```python
from build123d import *

# Parameters (mm, degrees)
F0_W          = 75.9948119521
F0_H          = 111.8377298117
F0_R          = 4.7655494626
F0_R_2        = 4.8016385214
F1_DEPTH      = 39.116
F2_R          = 25.2095031521
F2_R_2        = 17.6279340775
F3_DEPTH      = 50.8
F3_DEPTH_BACK = 50.8
F4_R          = 17.506739517
F5_DEPTH      = 77.978
F5_DEPTH_BACK = 76.962
F6_W          = 38.5849960148
F6_H          = 51.1202197522
F7_DEPTH      = 50.8
F7_DEPTH_BACK = 50.8


with BuildPart() as f1:
    # F0 (on Front) → F1 (new body)
    with BuildSketch(Plane.XZ):
        Rectangle(F0_W, F0_H)
        with Locations((0, -46.5174391866)):
            Circle(F0_R, mode=Mode.SUBTRACT)
        with Locations((0, 47.8884801269)):
            Circle(F0_R_2, mode=Mode.SUBTRACT)
    extrude(amount=-F1_DEPTH)

    # F2 (on Right) → F3 (join, two sides)
    with BuildSketch(Plane.YZ) as f3_sk:
        Circle(F2_R)
        Circle(F2_R_2, mode=Mode.SUBTRACT)
    extrude(amount=F3_DEPTH)
    extrude(f3_sk.sketch, amount=-F3_DEPTH_BACK)

    # F4 (on Right) → F5 (cut, two sides)
    with BuildSketch(Plane.YZ) as f5_sk:
        Circle(F4_R)
    extrude(amount=-F5_DEPTH, mode=Mode.SUBTRACT)
    extrude(f5_sk.sketch, amount=F5_DEPTH_BACK, mode=Mode.SUBTRACT)

    # F6 (on Right) → F7 (cut, two sides)
    with BuildSketch(Plane.YZ) as f7_sk:
        with Locations((-19.2924980074, 9.313e-07)):
            Rectangle(F6_W, F6_H)
    extrude(amount=-F7_DEPTH, mode=Mode.SUBTRACT)
    extrude(f7_sk.sketch, amount=F7_DEPTH_BACK, mode=Mode.SUBTRACT)


solid = f1.part
```
Read the model definition and answer for the solid it produces. Units are mm, in the model's axes. A direction names the side the tool comes from. Coordinates: 2 decimals unless noted, no trailing zeros. Loops run counter-clockwise (first coordinate to the right, second up) from the corner with the lowest first, then second, coordinate; pieces in that order, holes last. Notation, with made-up numbers: (49, 45.25) - (59, 45.25) arc R26 ccw to (59, 78.25) - close; hole circle Ø7 at (19, -24.5). An arc over 180 degrees is marked (long way). Answer in a Markdown table with one row per item.
1. Find section D-D, the plane x = -26. Write down the section's boundary in (y, z), then the cut area to 3 significant figures.
Conclusion:
| item | result |
|---|---|
| outline | (0, -55.92) - (39.12, -55.92) - (39.12, 55.92) - (0, 55.92) - (0, 17.51) arc R17.51 cw to (0, -17.51) - close |
| area | 3,890 mm² |
2. Straight lines are drawn through the part: line 1 (Z direction, x = 0, y = 24); line 2 (Z direction, x = 0, y = 10); line 3 (X direction, y = 38, z = 39). For each, find the intervals that lie inside material, in ascending order.
Conclusion:
| item | result |
|---|---|
| line 1 | z = -55.92 to -51.28, -41.75 to 43.09, 52.69 to 55.92 |
| line 2 | z = -55.92 to -51.28, -41.75 to -14.37, 14.37 to 43.09, 52.69 to 55.92 |
| line 3 | x = -38 to 38 |
3. Which of the six approach directions +Z, -Z, +X, -X, +Y, -Y give full straight-line access (tool end or side, diameter ignored) to faces 1 (the face through (44.309, 25.203, -0.554)), 2 (the face through (-44.309, 17.624, -0.388)), 3 (the face through (-37.997, 28, -1))?
Conclusion:
| item | result |
|---|---|
| face 1 | +X, +Y |
| face 2 | -X, -Y |
| face 3 | -X, +Y |
4. Given pin 1 (8 mm diameter, centred on x = 37.5, z = 1.5, fed in from -Y); pin 2 (4 mm diameter, centred on x = 9, z = -4, fed in from -Y); pin 3 (4 mm diameter, centred on y = 35, z = -10, fed in from -X); pin 4 (12 mm diameter, centred on y = 21, z = 19.5, fed in from -X), each flat-ended and moving along its own axis, determine where each tip first touches the part or whether it passes through.
Conclusion:
| item | result |
|---|---|
| pin 1 | stops at y = 16.62 |
| pin 2 | stops at y = 16.45 |
| pin 3 | stops at x = -38 |
| pin 4 | stops at x = -50.8 |
5. Find section C-C, the plane z = 0. Write down the section's boundary in (x, y).
Conclusion:
| item | result |
|---|---|
| outline | (-50.8, 17.63) - (-38, 17.63) - (-38, 17.51) - (38, 17.51) - (38, 17.63) - (50.8, 17.63) - (50.8, 25.21) - (38, 25.21) - (38, 39.12) - (-38, 39.12) - (-38, 25.21) - (-50.8, 25.21) - close |
6. Find section A-A, the plane x = 0. Write down the section's boundary in (y, z).
Conclusion:
| item | result |
|---|---|
| outline | (0, -55.92) - (39.12, -55.92) - (39.12, -51.28) - (0, -51.28) - close; (0, -41.75) - (39.12, -41.75) - (39.12, 43.09) - (0, 43.09) - (0, 17.51) arc R17.51 cw to (0, -17.51) - close; (0, 52.69) - (39.12, 52.69) - (39.12, 55.92) - (0, 55.92) - close |
7. Find section B-B, the plane y = 12.5. Write down the section's boundary in (x, z).
Conclusion:
| item | result |
|---|---|
| outline | (-50.8, -21.89) - (-38, -21.89) - (-38, -55.92) - (38, -55.92) - (38, -21.89) - (50.8, -21.89) - (50.8, -12.43) - (38, -12.43) - (38, -12.26) - (-38, -12.26) - (-38, -12.43) - (-50.8, -12.43) - close; (-50.8, 12.43) - (-38, 12.43) - (-38, 12.26) - (38, 12.26) - (38, 12.43) - (50.8, 12.43) - (50.8, 21.89) - (38, 21.89) - (38, 55.92) - (-38, 55.92) - (-38, 21.89) - (-50.8, 21.89) - close; hole circle Ø9.6 at (0, 47.89); hole circle Ø9.53 at (0, -46.52) |
8. Determine the mould class of faces 4 (the face through (-50.8, 18, 0)), 5 (the face through (-0.62, 19.284, -41.792)), 6 (the face through (44.309, 17.624, -0.388)), 7 (the face through (-1.04, 19.28, 43.2)) for opening direction X: +X half, -X half, draft (parallel to the pull), parting line (faces both ways), or undercut.
Conclusion:
| item | result |
|---|---|
| face 4 | -X half |
| face 5 | undercut |
| face 6 | draft |
| face 7 | undercut |
